```python
from build123d import *

# Parameters (mm, degrees)
SKETCH1_W           = 30
SKETCH1_H           = 30
BOSS_EXTRUDE1_DEPTH = 25
SKETCH2_W           = 20
SKETCH2_H           = 20
CUT_EXTRUDE1_DEPTH  = 20
CUT_EXTRUDE2_DEPTH  = 43
SKETCH4_W           = 30
SKETCH4_H           = 28.284271248
SKETCH4_W_2         = 10
SKETCH4_H_2         = 15
BOSS_EXTRUDE2_DEPTH = 2
SKETCH5_R           = 10.5
CUT_EXTRUDE4_DEPTH  = 5
SKETCH6_R           = 5
CUT_EXTRUDE6_DEPTH  = 5
SKETCH7_R           = 6.5
SKETCH7_R_2         = 5
CUT_EXTRUDE7_DEPTH  = 3.5


with BuildPart() as part:
    # Sketch1 → Boss-Extrude1 (new body)
    with BuildSketch(Plane(origin=(0, 0, 0), x_dir=(0, 1, 0), z_dir=(0, 0, 1))):
        Rectangle(SKETCH1_W, SKETCH1_H)
    extrude(amount=BOSS_EXTRUDE1_DEPTH)

    # Sketch2 → Cut-Extrude1 (cut)
    with BuildSketch(Plane.XY.offset(25)):
        Rectangle(SKETCH2_W, SKETCH2_H)
    extrude(amount=-CUT_EXTRUDE1_DEPTH, mode=Mode.SUBTRACT)

    # Sketch3 → Cut-Extrude2 (cut)
    with BuildSketch(Plane.YZ.offset(15)):
        Polygon((15, 25), (-10, 25), (10, 5), (15, 5), align=None)
    extrude(amount=-CUT_EXTRUDE2_DEPTH, mode=Mode.SUBTRACT)

    # Sketch4 → Boss-Extrude2 (add)
    with BuildSketch(Plane(origin=(0, 7.5, 7.5), x_dir=(-1, 0, 0), z_dir=(0, 0.7071067811865477, 0.7071067811865475))):
        with Locations((0, 10.606601718)):
            Rectangle(SKETCH4_W, SKETCH4_H)
        with Locations((0, 10.606601718)):
            Rectangle(SKETCH4_W_2, SKETCH4_H_2, mode=Mode.SUBTRACT)
    extrude(amount=-BOSS_EXTRUDE2_DEPTH)

    # Sketch5 → Cut-Extrude4 (cut)
    with BuildSketch(Plane(origin=(0, 0, 0), x_dir=(1, 0, 0), z_dir=(0, 0, -1))):
        with Locations(Location((0, 0, 0), (0, 0, 180))):
            Circle(SKETCH5_R)
    extrude(amount=-CUT_EXTRUDE4_DEPTH, mode=Mode.SUBTRACT)

    # Sketch6 → Cut-Extrude6 (cut)
    with BuildSketch(Plane.XZ.offset(15)):
        with Locations(Location((0, 15, 0), (0, 0, 270))):
            Circle(SKETCH6_R)
    extrude(amount=-CUT_EXTRUDE6_DEPTH, mode=Mode.SUBTRACT)

    # Sketch7 → Cut-Extrude7 (cut)
    with BuildSketch(Plane.XZ.offset(15)):
        with Locations(Location((0, 15, 0), (0, 0, 270))):
            Circle(SKETCH7_R)
        with Locations(Location((0, 15, 0), (0, 0, 270))):
            Circle(SKETCH7_R_2, mode=Mode.SUBTRACT)
    extrude(amount=-CUT_EXTRUDE7_DEPTH, mode=Mode.SUBTRACT)


solid = part.part
```
Could you check a few things on this model? Use its own coordinates, in mm. A direction names the side the tool comes from. Coordinates: 2 decimals unless noted, no trailing zeros. Order: outer loops, then holes, each group sorted by start corner. A loop starts at its lowest first (then second) coordinate and runs counter-clockwise, first axis right, second up. Notation, with made-up numbers: M 14,20 L 48,20 A16 cw 48,27 Z; hole C 21,-5.75 d3. An arc over 180 degrees is marked long. Use one line per item in the form item = value. Start each with the question number.
1. On a 3-axis mill with a long thin cutter (end or side, diameter ignored), from which of +Z, -Z, +X, -X, +Y, -Y can I reach the whole of each face in a straight line? I mean faces 4 (the flat face through (0, 12, 5)), 5 (the cylindrical face through (0, -11, 20)), 6 (the flat face through (6.807, -1.534, 13.706)), 7 (the flat face through (0.07, 4.606, 8.999)). Say none if no direction works.
2. Suppose I cut it at B-B on y = 0. Write out the boundary of the cut face in (x, z), then the cut area to 3 significant figures.
3. Please list where these lines run through material, in increasing order: line 1 (X direction, y = -5.75, z = 13.75); line 2 (Y direction, x = 0, z = 2.1).
4. We'd pull the mould along Y, two halves only. Please class faces 1 (the flat face through (-10, -4, 0)), 2 (the flat face through (-8, -8, 5)), 3 (the flat face through (-5, -11.5, 13)): +Y half, -Y half, draft (parallel to the pull), parting line (faces both ways), or undercut.
5. Suppose I cut it at D-D on z = 7. Write out the boundary of the cut face in (x, y).
6. For pin 1 (7.5 mm diameter, centred on x = 5.5, y = -7.5, fed in from +Z); pin 2 (1 mm diameter, centred on x = -4, y = -7, fed in from +Z); pin 3 (1 mm diameter, centred on x = 9, z = 21.5, fed in from +Y); pin 4 (1.4 mm diameter, centred on x = 3.5, y = 9, fed in from -Z), each with a flat end and sliding along its axis, tell me the tip position at first contact or that it passes through.
7. Suppose I cut it at A-A on x = 0. Write out the boundary of the cut face in (y, z).
8. Suppose I cut it at C-C on z = 13.75. Write out the boundary of the cut face in (x, y), then the cut area to 3 significant figures.
Geometry says:
q1.face_4 = +Z, +X, -X, +Y
q1.face_5 = -Y
q1.face_6 = none
q1.face_7 = +Z
q2.outline = M -15,0 L -10.5,0 L -10.5,5 L -10,5 L -10,12.17 L -5,12.17 L -5,15 L -15,15 Z; M 5,12.17 L 10,12.17 L 10,5 L 10.5,5 L 10.5,0 L 15,0 L 15,15 L 5,15 Z
q2.area = 173 mm^2
q3.line_1 = -15 to -10, 10 to 15
q3.line_2 = -15 to -10.5, 10.5 to 15
q4.face_1 = draft
q4.face_2 = undercut
q4.face_3 = -Y half
q5.outline = M -15,-15 L 15,-15 L 15,8 L -15,8 Z; hole M -10,-10 L 10,-10 L 10,5.17 L -10,5.17 Z
q6.pin_1 = 25
q6.pin_2 = 22.5
q6.pin_3 = -6
q6.pin_4 = 5
q7.outline = M -15,0 L -10.5,0 L -10.5,5 L -10,5 L -10,10 L -11.5,10 L -11.5,8.5 L -15,8.5 Z; M -15,21.5 L -11.5,21.5 L -11.5,20 L -10,20 L -10,22.17 L -6.72,18.89 L -5.3,20.3 L -10,25 L -15,25 Z; M 3.89,8.28 L 7.17,5 L 10,5 L 5.3,9.7 Z; M 10.5,0 L 15,0 L 15,5 L 10.5,5 Z
q8.outline = M -15,-15 L -6.38,-15 L -6.38,-11.5 L -4.84,-11.5 L -4.84,-10 L -10,-10 L -10,-1.58 L -5,-1.58 L -5,1.25 L -15,1.25 Z; M 4.84,-11.5 L 6.38,-11.5 L 6.38,-15 L 15,-15 L 15,1.25 L 5,1.25 L 5,-1.58 L 10,-1.58 L 10,-10 L 4.84,-10 Z
q8.area = 232 mm^2
